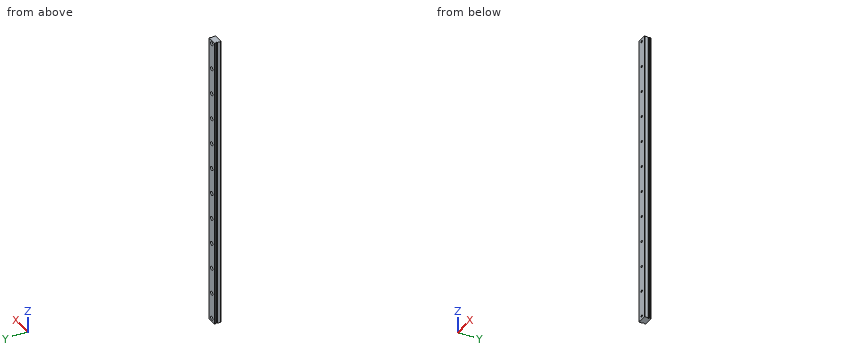
from build123d import *

# Parameters (mm, degrees)
EXTRUDE_1_DEPTH           = 450
HOLE_WIZARD_1_D           = 3.2
HOLE_WIZARD_1_CBORE_D     = 6
HOLE_WIZARD_1_CBORE_DEPTH = 4.5


with BuildPart() as part:
    # 草图1 → 凸台-拉伸1 (new body)
    with BuildSketch(Plane.XY):
        Polygon((-3.269035533, 4.949238579), (10.730964467, 4.949238579), (11.230964467, 4.449238579), (11.230964467, 2.317517259), (10.086764657, 1.783377919), (10.086764657, 0.983377919), (11.230964467, 0.449238579), (11.230964467, -4.550761421), (10.730964467, -5.050761421), (-3.269035533, -5.050761421), (-3.769035533, -4.550761421), (-3.769035533, 0.449238579), (-2.624835723, 0.983377919), (-2.624835723, 1.783377919), (-3.769035533, 2.317517259), (-3.769035533, 4.449238579), align=None)
    extrude(amount=-EXTRUDE_1_DEPTH)

    # 孔1 (through all)
    with Locations(Plane(origin=(3.730964467, 4.949238579, -445), x_dir=(0, 0, 1), z_dir=(0, 1, 0))):
        with Locations((0, 0), (40, 0), (80, 0), (120, 0), (160, 0), (200, 0), (240, 0), (280, 0), (320, 0), (360, 0), (400, 0), (440, 0)):
            CounterBoreHole(HOLE_WIZARD_1_D / 2, HOLE_WIZARD_1_CBORE_D / 2, HOLE_WIZARD_1_CBORE_DEPTH)


solid = part.part
Design review of the part built by this model. Coordinates are the model's own, in mm. Coordinates: 2 decimals unless noted, no trailing zeros. Write each loop counter-clockwise with the first axis right and the second up, starting at its lowest first coordinate (ties: lowest second). Pieces come first, ordered by that corner, then holes. Notation, with made-up numbers: (25.5, 11) - (65.5, 11) arc R29 ccw to (65.5, 36) - close; hole circle Ø9 at (19, 74.5). An arc over 180 degrees is marked (long way). Use one line per item in the form item = value.
Q1. For probe 1 along X at (y, z) = (2.95, -125); probe 2 along X at (y, z) = (-0.25, -245); probe 3 along Y at (x, z) = (6.25, -165.5), list the stretches that pass through material, from the lowest coordinate up.
Taken from the geometry:
probe_1 = -3.77 to 0.73, 6.73 to 11.23
probe_2 = -3.77 to 2.13, 5.33 to 11.23
probe_3 = -5.05 to 0.45
Q2. Insertion check: pin 1 Ø1.8 at (x, z) = (3.5, -404) entering from +Y; pin 2 Ø0.9 at (y, z) = (1.5, -150.5) entering from +X. Each pin has a flat end and moves straight along its axis. Give the tip position at first contact, or say it passes through.
Taken from the geometry:
pin_1 = 0.45
pin_2 = 10.44
Q3. Consider section A-A (z = -273). Write out the cut boundary in (x, y).
Taken from the geometry:
outline = (-3.77, -4.55) - (-3.27, -5.05) - (10.73, -5.05) - (11.23, -4.55) - (11.23, 0.45) - (10.09, 0.98) - (10.09, 1.78) - (11.23, 2.32) - (11.23, 4.45) - (10.73, 4.95) - (-3.27, 4.95) - (-3.77, 4.45) - (-3.77, 2.32) - (-2.62, 1.78) - (-2.62, 0.98) - (-3.77, 0.45) - close
